Source: three-view drawing plus pictorial views. Frame: mm from the lowest corner of the part. Round coordinates to 2 decimals unless told otherwise and drop trailing zeros. Answer as CSV lines item,"result".
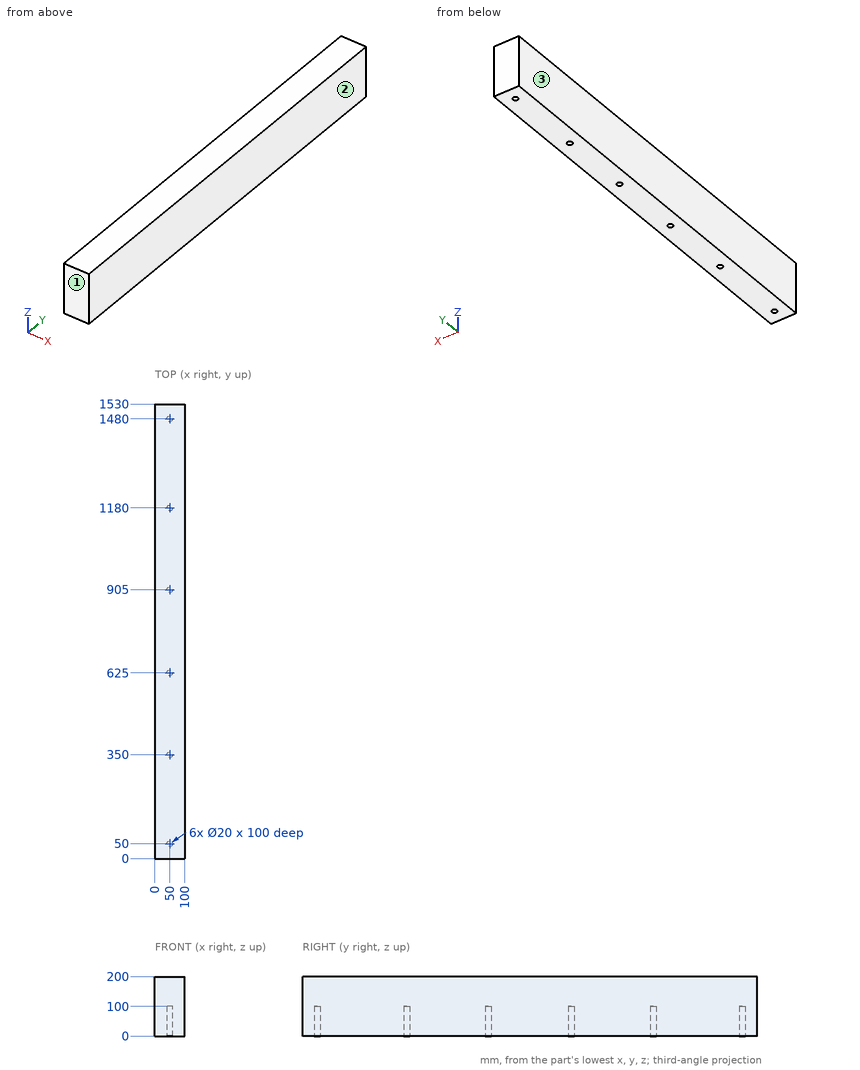
1. Mould query, pull axis X, two halves, no side actions, for the marked faces 1, 2 and 3. Classes: released by +X, released by -X, zero draft, split by the parting line, or undercut.
Results below:
face 1,"zero draft"
face 2,"released by +X"
face 3,"released by -X"
2. Line query: L1, parallel to X at y = 1180, z = 50. Output: solid intervals per line, ascending. Write a range as [from, to].
Results below:
L1,"[0, 40], [60, 100]"
3. Pin query (flat end, axial travel): pin 1 (10 mm diameter, centred on x = 46.5, y = 622.5, fed in from -Z). Return the tip coordinate at first contact, or that it passes through.
Results below:
pin 1,"z = 100"
